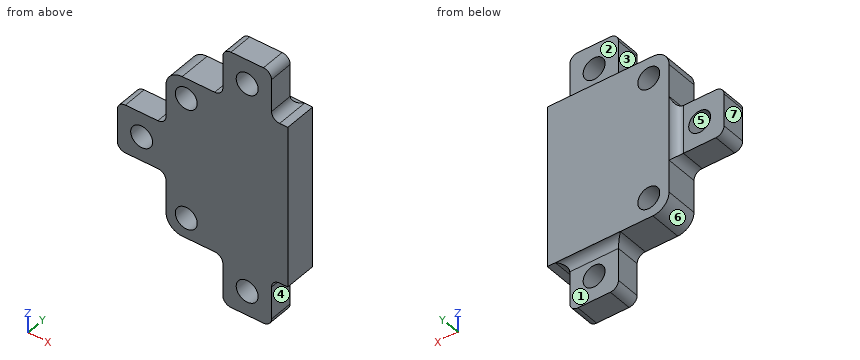
Autodesk Inventor part; units mm, degrees
ref_plane "YZ Plane" through (0, 0, 0) normal (1, 0, 0) x (0, 1, 0)
ref_plane "XZ Plane" through (0, 0, 0) normal (0, 1, 0) x (-1, 0, 0)
ref_plane "XY Plane" through (0, 0, 0) normal (0, 0, 1) x (1, 0, 0)
sketch "Эскиз1" plane through (0, 0, 0) normal (0, 1, 0) x (-1, 0, 0)
  line L0 (10, -10) -> (10, 10)
  line L1 (10, 0) -> (-10, 0) construction
  line L2 (0, -10) -> (0, 10) construction
  line L3 (10, -10) -> (9, -10) construction
  line L4 (10, -9) -> (10, -10) construction
  circle A0 centre (7.5, -7.5) radius 1.35
  circle A1 centre (7.5, 7.5) radius 1.35
  line L5 (10, -10) -> (-5, -10)
  line L6 (10, 10) -> (-5, 10)
  line L7 (-5, 10) -> (-5, -10)
  point P0 (0, 0)
  point P1 (0, 0)
  point P2 (0, 0)
  dimension "d16" = 2.7
  dimension "d17" = 2.7
  dimension "d25" = 15
  dimension "d26" = 15
extrude "Выдавливание1" add sketch "Эскиз1" along normal blind 4 contours L5 L7 L6 L0 | A0 | A1
sketch "Эскиз2" plane through (0, 0, 0) normal (0, -1, 0) x (1, 0, 0)
  line L0 (0, -10) -> (2.5, -10) construction
  line L1 (0, -10) -> (-3, -10)
  line L2 (-3, -10) -> (-3, -16)
  line L3 (-3, -16) -> (0, -16)
  line L4 (-3, -16) -> (3, -16)
  line L5 (3, -16) -> (3, -10)
  line L6 (3, -10) -> (-3, -10)
  line L7 (-3, -10) -> (-3, -16)
  line L8 (-10, -10) -> (-10, 10) construction
  line L9 (-10, 0) -> (5, 0) construction
  line L10 (5, 10) -> (5, -10) construction
  line L11 (0, 10) -> (2.5, 10) construction
  line L12 (0, 15) -> (0, 10) construction
  line L13 (0, 10) -> (-3, 10)
  line L14 (-3, 16) -> (0, 16)
  line L15 (-3, 16) -> (3, 16)
  line L16 (3, 16) -> (3, 10)
  line L17 (3, 10) -> (-3, 10)
  line L18 (5, -10) -> (5, 10) construction
  line L19 (-3, 16) -> (-3, 10)
  line L20 (-10, 10) -> (5, 10) construction
  line L21 (-2.5, 0) -> (-10, 10) construction
  line L22 (-10, 0) -> (-16, 0) construction
  line L23 (-16, 0) -> (-16, -3) construction
  line L24 (-16, -3) -> (-10, -3) construction
  line L25 (-10, -3) -> (-10, 0) construction
  line L26 (-10, -3) -> (-16, -3)
  line L27 (-16, -3) -> (-16, 3)
  line L28 (-16, 3) -> (-10, 3)
  line L29 (-10, 3) -> (-10, -3)
  circle A0 centre (-13, 0) radius 1.35
  circle A1 centre (0, 13) radius 1.35
  circle A2 centre (0, -13) radius 1.35
  point P0 (-2.5, -10)
  dimension "d30" = 6
  dimension "d31" = 6
  dimension "d33" = 6
  dimension "d34" = 3
  dimension "d35" = 6
  dimension "d39" = 2.7
  dimension "d40" = 2.7
  dimension "d41" = 2.7
extrude "Выдавливание2" cut sketch "Эскиз1" along normal blind 4 contours A0 | A1
fillet "Сопряжение3" radius 2 2 edges at (-10, 2, 10) (-10, 2, -10)
extrude "Выдавливание4" add sketch "Эскиз2" against normal blind 3
fillet "Сопряжение6" radius 1 15 edges at (3, 1.5, 16) (3, 1.5, 10) (-3, 1.5, 16) (-3, 1.5, 10) (0, 3, 10) (-10, 1.5, 3) (-16, 1.5, 3) (-16, 1.5, -3) (-10, 1.5, -3) (-10, 3, 0) (-3, 1.5, -10) (0, 3, -10) (-3, 1.5, -16) (3, 1.5, -16) (3, 1.5, -10)
properties part number "крепление_RGB"
Geometry check sheet. Reference: the model listing, model coordinates, mm. Face numbers are marked on the shaded views. A direction names the side the tool comes from. Give positions to 0.01 mm unless a question says otherwise; leave off trailing zeros. Order: outer loops, then holes, each group sorted by start corner. A loop starts at its lowest first (then second) coordinate and runs counter-clockwise, first axis right, second up.
1. Access from +Z, -Z, +X, -X, +Y, -Y to the whole of each face (thin tool, end or side, straight path). Record for the marked faces 1, 2, 3 and 4.
Completed:
face 1: -Z, +X, -X, +Y
face 2: +Z, +X, -X, +Y
face 3: +Z, -X, +Y, -Y
face 4: -Z, +X, +Y, -Y
2. Sectioned sample at C-C (x = 0). State how many separate pieces and enclosed holes the cut face has, then the cut area to 3 significant figures.
Completed:
separate pieces: 3
enclosed holes: 0
area: 100 mm2
3. Scan lines: line 1 (Z direction, x = 0, y = 1.2); line 2 (Z direction, x = -8.5, y = 3.5); line 3 (Z direction, x = -5.5, y = 0.8). Record each from-to range of solid material in increasing order.
Completed:
line 1: z = -16 to -14.35, -11.65 to 11.65, 14.35 to 16
line 2: z = -9.94 to -8.41, -6.59 to 6.59, 8.41 to 9.94
line 3: z = -10 to 10
4. Sectioned sample at B-B (x = -13). Record the boundary of the cut face in (y, z).
Completed:
outline: (0, -3) - (3, -3) - (3, -1.35) - (0, -1.35) - close; (0, 1.35) - (3, 1.35) - (3, 3) - (0, 3) - close
5. Depth check by flat-ended pin: pin 1 (0.9 mm diameter, centred on y = 1, z = -12, fed in from +X); pin 2 (5.5 mm diameter, centred on x = -12.5, z = -1, fed in from +Y); pin 3 (1.5 mm diameter, centred on y = 1, z = -13, fed in from -X); pin 4 (1.5 mm diameter, centred on x = -13, y = 2, fed in from +Z). Enter the tip coordinate at first touch or a pass-through.
Completed:
pin 1: stops at x = 3
pin 2: stops at y = 4
pin 3: stops at x = -3
pin 4: stops at z = 3
6. Draft check along Z on the marked faces 5, 6 and 7. Enter one of: pulls with the +Z half, pulls with the -Z half, needs draft (parallel to the pull), parting line crosses it, or undercut.
Completed:
face 5: undercut
face 6: pulls with the -Z half
face 7: needs draft
